Can you work these out from the model? Positions are in its coordinate system, mm. A direction names the side the tool comes from. Round coordinates to 2 decimals unless told otherwise and drop trailing zeros. Write each loop counter-clockwise with the first axis right and the second up, starting at its lowest first coordinate (ties: lowest second). Pieces come first, ordered by that corner, then holes. Notation, with made-up numbers: M 12,69 L 52,69 A13 cw 52,93 Z; hole C 39,66 d8. An arc over 180 degrees is marked long. Answer as a JSON object with one key per item and string values. Group by question number.
1) I'm going to push a flat-ended pin straight in: pin 1 Ø4 at (y, z) = (-8, 3.5) entering from -X. Where does the tip first touch, or does it pass through?
2) Suppose I cut it at B-B, the plane y = -16. Write out the boundary of the cut face in (x, z), and give its area (3 significant figures).
3) Please list where these lines run through material, in increasing order: L1, parallel to Z at x = 0, y = -23; L2, parallel to Z at x = 0.05, y = -15; L3, parallel to Y at x = 0.3, z = 7.5. Write a range as [from, to].
4) Suppose I cut it at A-A, the plane x = 0. Write out the boundary of the cut face in (y, z).
5) On a 3-axis mill with a long thin cutter (end or side, diameter ignored), from which of +Z, -Z, +X, -X, +Y, -Y can I reach the whole of each face in a straight line? I mean faces 3 (the cylindrical face through (0.108, -7.605, 0.488)), 4 (the flat face through (0, -15, 0)), 5 (the cylindrical face through (0.5, -15, 3.8)). Say none if no direction works.
6) If we mould it in two halves opening along X, with no side actions, what happens to faces 1 (the flat face through (0, -15, 7.5)), 2 (the cylindrical face through (0, -31, 8))? For each: +X half, -X half, draft (parallel to the pull), parting line (faces both ways), or undercut.
Autodesk Inventor part; units mm, degrees
ref_plane "YZ Plane" through (0, 0, 0) normal (1, 0, 0) x (0, 1, 0)
ref_plane "XZ Plane" through (0, 0, 0) normal (0, 1, 0) x (-1, 0, 0)
ref_plane "XY Plane" through (0, 0, 0) normal (0, 0, 1) x (1, 0, 0)
sketch "Skizze1" plane through (0, 0, 0) normal (1, 0, 0) x (0, 1, 0)
  line L0 (0, 0) -> (-15, 0)
  line L1 (-15, 0) -> (-15, 7.5)
  line L2 (-15, 7.5) -> (-45.667, 7.5)
  dimension "d0" = 15
  dimension "d1" = 7.5
sketch "Skizze2" plane through (0, 0, 0) normal (0, 1, 0) x (-1, 0, 0)
  circle A0 centre (0, 0) radius 0.5
  dimension "d2" = 1
sweep "Sweeping1" add profiles "Skizze2" path "Skizze1"
sketch "Skizze3" plane through (0, 0, 0) normal (1, 0, 0) x (0, 1, 0)
  line L0 (-14.5, 0.5) -> (-14.5, 8)
  line L1 (-15.5, -0.5) -> (-15.5, 7)
  line L2 (-13.783, 17.8624) -> (-5.8155, 9.8948)
  line L3 (-5.8155, 9.8948) -> (-11.6052, 4.1052)
  line L4 (-11.6052, 4.1052) -> (-19.5727, 12.0727)
  line L5 (-19.5727, 12.0727) -> (-13.783, 17.8624)
  line L6 (-13.783, 17.8624) -> (-11.6052, 4.1052) construction
  line L7 (-5.8155, 9.8948) -> (-19.5727, 12.0727) construction
  line L8 (-13.783, 17.8624) -> (-2.5152, 17.8624) construction
  line L9 (-14.4975, -10.7606) -> (-21.8094, -3.4488)
  line L10 (-21.8094, -3.4488) -> (-16.6803, 1.6803)
  line L11 (-16.6803, 1.6803) -> (-9.3684, -5.6316)
  line L12 (-9.3684, -5.6316) -> (-14.4975, -10.7606)
  line L13 (-14.4975, -10.7606) -> (-16.6803, 1.6803) construction
  line L14 (-21.8094, -3.4488) -> (-9.3684, -5.6316) construction
  point P0 (0, 0)
  point P1 (-12.6941, 10.9838)
  point P2 (-15.5889, -4.5402)
  dimension "d5" = 45
extrude "Extrusion1" cut sketch "Skizze3" along normal through all both and the other way through all
properties part number "00_Beam_Stairs_7.5mm"
Results:
{
 "1": {"pin 1": "through"},
 "2": {"outline": "C 0,7.5 d1", "area": "0.785 mm^2"},
 "3": {"L1": "[7, 8]", "L2": "[0, 7.5]", "L3": "[-45.67, -15]"},
 "4": {"outline": "M -45.67,7 L -15.5,7 L -15.5,0.5 L -14.5,-0.5 L 0,-0.5 L 0,0.5 L -14.5,0.5 L -14.5,7 L -15.5,8 L -45.67,8 Z"},
 "5": {"face 3": "+Y", "face 4": "-Z, +X, -X, -Y", "face 5": "none"},
 "6": {"face 1": "draft", "face 2": "parting line"}
}
